Can you work these out from the model? Positions are in its coordinate system, mm. Round coordinates to 2 decimals unless told otherwise and drop trailing zeros. Write each loop counter-clockwise with the first axis right and the second up, starting at its lowest first coordinate (ties: lowest second). Pieces come first, ordered by that corner, then holes. Notation, with made-up numbers: M 83.5,47 L 95.5,47 A28 cw 95.5,76 Z; hole C 43.25,51 d11. An arc over 180 degrees is marked long. Answer in a Markdown table with one row per item. Add a question column.
(1) I'm going to push flat-ended pins straight in: pin 1 (1 mm diameter, centred on x = 91.5, z = 2, fed in from +Y); pin 2 (1.5 mm diameter, centred on x = 146, z = 1, fed in from +Y); pin 3 (5 mm diameter, centred on x = 101.5, y = 0.5, fed in from -Z); pin 4 (0.6 mm diameter, centred on x = 40.5, y = 3, fed in from -Z). Where does each tip first touch, or does it pass through?
(2) Suppose I cut it at A-A, the plane z = 0. Write out the boundary of the cut face in (x, y).
(3) If I drill on probe 1 along X at (y, z) = (3.25, 0); probe 2 along X at (y, z) = (4.25, -1.5); probe 3 along Y at (x, z) = (13, 0.5), over which ranges is the centre line in solid material (lowest first)?
(4) Suppose I cut it at B-B, the plane x = 165. Write out the boundary of the cut face in (y, z).
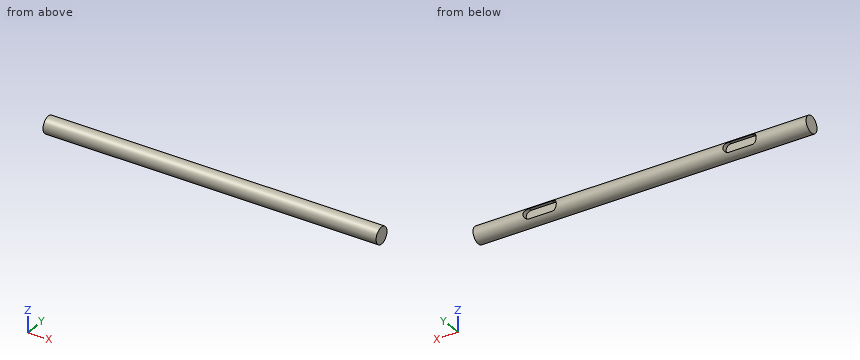
from build123d import *

# Parameters (mm, degrees)
SKETCH_1_R          = 5
EXTRUDE_1_DEPTH     = 100
CUT_EXTRUDE_1_DEPTH = 3
SKETCH_3_R          = 5
EXTRUDE_2_DEPTH     = 100
CUT_EXTRUDE_2_DEPTH = 3


with BuildPart() as part:
    # 草图1 → 凸台-拉伸1 (new body)
    with BuildSketch(Plane(origin=(0, 0, 0), x_dir=(0, 0, -1), z_dir=(1, 0, 0))):
        Circle(SKETCH_1_R)
    extrude(amount=EXTRUDE_1_DEPTH)

    # 草图2 → 切除-拉伸1 (cut)
    with BuildSketch(Plane(origin=(0, 5, 0), x_dir=(1, 0, 0), z_dir=(0, 1, 0))):
        with BuildLine():
            Line((33, 3), (47, 3))
            ThreePointArc((47, 3), (50, 0), (47, -3))
            Line((47, -3), (33, -3))
            ThreePointArc((33, -3), (30, 0), (33, 3))
        make_face()
    extrude(amount=-CUT_EXTRUDE_1_DEPTH, mode=Mode.SUBTRACT)

    # 草图3 → 凸台-拉伸2 (add)
    with BuildSketch(Plane(origin=(100, 0, 0), x_dir=(0, 0, -1), z_dir=(1, 0, 0))):
        Circle(SKETCH_3_R)
    extrude(amount=EXTRUDE_2_DEPTH)

    # 草图4 → 切除-拉伸2 (cut)
    with BuildSketch(Plane(origin=(0, 5, 0), x_dir=(1, 0, 0), z_dir=(0, 1, 0))):
        with BuildLine():
            Line((153, 3), (167, 3))
            ThreePointArc((167, 3), (170, 0), (167, -3))
            Line((167, -3), (153, -3))
            ThreePointArc((153, -3), (150, 0), (153, 3))
        make_face()
    extrude(amount=-CUT_EXTRUDE_2_DEPTH, mode=Mode.SUBTRACT)


solid = part.part
Calculated:
| question | item | result |
|---|---|---|
| 1 | pin 1 | y = 4.77 |
| 1 | pin 2 | y = 4.99 |
| 1 | pin 3 | z = -5 |
| 1 | pin 4 | z = -4.21 |
| 2 | outline | M 0,-5 L 200,-5 L 200,5 L 170,5 L 170,2 L 150,2 L 150,5 L 50,5 L 50,2 L 30,2 L 30,5 L 0,5 Z |
| 3 | probe 1 | 0 to 30, 50 to 150, 170 to 200 |
| 3 | probe 2 | 0 to 30.4, 49.6 to 150.4, 169.6 to 200 |
| 3 | probe 3 | -4.97 to 4.97 |
| 4 | outline | M 2,-3 L 2,3 L 4,3 A5 ccw long 4,-3 Z |
